For this review, take the finished solid that the model builds, in its own axes (mm). A direction names the side the tool comes from. Round coordinates to 2 decimals unless told otherwise and drop trailing zeros. Order: outer loops, then holes, each group sorted by start corner. A loop starts at its lowest first (then second) coordinate and runs counter-clockwise, first axis right, second up.
```python
from build123d import *

# Parameters (mm, degrees)
SKETCH1_W           = 40
SKETCH1_H           = 26
BOSS_EXTRUDE1_DEPTH = 1.5
SKETCH2_R           = 4
CUT_EXTRUDE1_DEPTH  = 3
SKETCH8_W           = 5
SKETCH8_H           = 3
BOSS_EXTRUDE7_DEPTH = 3
SKETCH9_W           = 5
SKETCH9_H           = 3
CUT_EXTRUDE2_DEPTH  = 3


with BuildPart() as part:
    # Sketch1 → Boss-Extrude1 (new body, symmetric)
    with BuildSketch(Plane(origin=(0, 0, 0), x_dir=(1, 0, 0), z_dir=(0, 1, 0))):
        Rectangle(SKETCH1_W, SKETCH1_H)
    extrude(amount=BOSS_EXTRUDE1_DEPTH, both=True)

    # Sketch2 → Cut-Extrude1 (cut)
    with BuildSketch(Plane.XZ.offset(1.5)):
        with Locations((10, 0)):
            Circle(SKETCH2_R)
    extrude(amount=-CUT_EXTRUDE1_DEPTH, mode=Mode.SUBTRACT)

    # Sketch8 → Boss-Extrude7 (add)
    with BuildSketch(Plane.ZY.offset(20)):
        with Locations((-7.5, 0)):
            Rectangle(SKETCH8_W, SKETCH8_H)
        with Locations((2.5, 0)):
            Rectangle(SKETCH8_W, SKETCH8_H)
    extrude(amount=BOSS_EXTRUDE7_DEPTH)

    # Sketch9 → Cut-Extrude2 (cut)
    with BuildSketch(Plane.XZ.offset(1.5)):
        with Locations((-17.5, -11.5)):
            Rectangle(SKETCH9_W, SKETCH9_H)
        with Locations((-7.5, -11.5)):
            Rectangle(SKETCH9_W, SKETCH9_H)
        with Locations((-17.5, 11.5)):
            Rectangle(SKETCH9_W, SKETCH9_H)
        with Locations((-7.5, 11.5)):
            Rectangle(SKETCH9_W, SKETCH9_H)
        with Locations((2.5, 11.5)):
            Rectangle(SKETCH9_W, SKETCH9_H)
        with Locations((12.5, 11.5)):
            Rectangle(SKETCH9_W, SKETCH9_H)
        with Locations((2.5, -11.5)):
            Rectangle(SKETCH9_W, SKETCH9_H)
        with Locations((12.5, -11.5)):
            Rectangle(SKETCH9_W, SKETCH9_H)
    extrude(amount=-CUT_EXTRUDE2_DEPTH, mode=Mode.SUBTRACT)


solid = part.part
```
Q1. Take a section at B-B, the plane z = 7.25. State the section outline as (x, y) points.
Q2. Wall thickness on line 1 (Z direction, x = 14.5, y = 1.2); line 2 (Z direction, x = 9.5, y = -1.25); line 3 (X direction, y = -1.25, z = -1): over which ranges is each line inside the solid? List them lowest first.
Q3. Mouldability with a two-part tool opening along X and no side actions: class faces 6 (the face through (-20, 0, 8)), 7 (the face through (17, 0, -13)), 8 (the face through (-10, 0, -12)) as +X half, -X half, draft (parallel to the pull), parting line (faces both ways), or undercut.
Q4. Take a section at A-A, the plane z = -1. State the section outline as (x, y) points, plus the area to 3 significant figures.
Q5. Clearance check with flat-ended pins moving along their axes: pin 1 (1.5 mm diameter, centred on y = 0.5, z = -11, fed in from -X); pin 2 (1.5 mm diameter, centred on x = -21.5, y = -0.5, fed in from -Z); pin 3 (0.9 mm diameter, centred on x = -17.5, y = -0.5, fed in from +Z). State where each tip first meets the part, or that it passes through.
Q6. Take a section at C-C, the plane x = 14.5. State the section outline as (y, z) points.
Q7. Tool access review of faces 1 (the face through (-10, 0, 11)), 2 (the face through (-15, 0, -12)), 3 (the face through (-21, 0, 5)), 4 (the face through (-20, 0, -2)), 5 (the face through (2, 0, -10)): name each direction out of +Z, -Z, +X, -X, +Y, -Y from which nothing blocks a thin tool from reaching the whole face with its end or side.
Working result:
1. outline: (-20, -1.5) - (20, -1.5) - (20, 1.5) - (-20, 1.5) - close
2. line 1: z = -10 to 10
2. line 2: z = -13 to -3.97, 3.97 to 13
2. line 3: x = -20 to 6.13, 13.87 to 20
3. face 6: -X half
3. face 7: draft
3. face 8: undercut
4. outline: (-20, -1.5) - (6.13, -1.5) - (6.13, 1.5) - (-20, 1.5) - close; (13.87, -1.5) - (20, -1.5) - (20, 1.5) - (13.87, 1.5) - close
4. area: 96.8 mm2
5. pin 1: stops at x = -15
5. pin 2: stops at z = -10
5. pin 3: stops at z = 10
6. outline: (-1.5, -10) - (1.5, -10) - (1.5, 10) - (-1.5, 10) - close
7. face 1: +Z, +Y, -Y
7. face 2: -Z, -X, +Y, -Y
7. face 3: +Z, -X, +Y, -Y
7. face 4: -X, +Y, -Y
7. face 5: -Z, +Y, -Y
